```python
from build123d import *

# Parameters (mm, degrees)
SKETCH011_W     = 19.6
SKETCH011_H     = 4.05
PAD007_DEPTH    = 1.7
SKETCH005_R     = 3.1
PAD004_DEPTH    = 4.3
SKETCH004_R     = 3.1
PAD003_DEPTH    = 4.3
PAD_DEPTH       = 5.5
SKETCH001_W     = 89.8
SKETCH001_H     = 9.3
POCKET_DEPTH    = 3.75
SKETCH006_R     = 3.1
PAD005_DEPTH    = 4.2
SKETCH010_R     = 1.6
POCKET002_DEPTH = 3.2
SKETCH008_R     = 3.1
PAD006_DEPTH    = 4.2
SKETCH009_R     = 1.6
POCKET001_DEPTH = 3.2


with BuildPart() as body006:
    # Sketch011 → Pad007 (new body)
    with BuildSketch(Plane.YZ.offset(97.7)):
        with Locations((9.8, 3.725)):
            Rectangle(SKETCH011_W, SKETCH011_H)
    extrude(amount=-PAD007_DEPTH)


with BuildPart() as body002:
    # Sketch005 → Pad004 (new body)
    with BuildSketch(Plane.YZ.offset(93.4)):
        with Locations((20.07, 3.1)):
            Circle(SKETCH005_R)
    extrude(amount=PAD004_DEPTH)


with BuildPart() as fusion:
    # Sketch004 → Pad003 (new body)
    with BuildSketch(Plane.YZ):
        with Locations((20.07, 3.1)):
            Circle(SKETCH004_R)
    extrude(amount=PAD003_DEPTH)

    # Fusion: union Body002
    add(body002.part)


with BuildPart() as cut:
    # Sketch → Pad (new body)
    with BuildSketch(Plane.XY):
        Polygon((0, 0), (97.7, 0), (97.7, 20.1), (93.4, 20.1), (93.4, 15), (4.3, 15), (4.3, 20.1), (0, 20.1), align=None)
    extrude(amount=PAD_DEPTH)

    # Sketch001 (on Face10 of Pad) → Pocket (cut)
    with BuildSketch(Plane.XY.offset(5.5)):
        with Locations((48.9, 8.15)):
            Rectangle(SKETCH001_W, SKETCH001_H)
    extrude(amount=-POCKET_DEPTH, mode=Mode.SUBTRACT)

    # Cut: cut Fusion
    add(fusion.part, mode=Mode.SUBTRACT)


with BuildPart() as fusion001:
    # Sketch006 → Pad005 (new body)
    with BuildSketch(Plane.YZ):
        with Locations((20.07, 3.1)):
            Circle(SKETCH006_R)
    extrude(amount=PAD005_DEPTH)

    # Sketch010 (on Face2 of Pad005) → Pocket002 (cut)
    with BuildSketch(Plane(origin=(0, 0, 0), x_dir=(0, 1, 0), z_dir=(-1, 0, 0))):
        with Locations((20.07, -3.1)):
            Circle(SKETCH010_R)
    extrude(amount=-POCKET002_DEPTH, mode=Mode.SUBTRACT)

    # Fusion001: union Cut
    add(cut.part)


with BuildPart() as cut001:
    # Sketch008 → Pad006 (new body)
    with BuildSketch(Plane.YZ.offset(97.7)):
        with Locations((20.07, 3.1)):
            Circle(SKETCH008_R)
    extrude(amount=-PAD006_DEPTH)

    # Sketch009 (on Face2 of Pad006) → Pocket001 (cut)
    with BuildSketch(Plane.YZ.offset(97.7)):
        with Locations((20.07, 3.1)):
            Circle(SKETCH009_R)
    extrude(amount=-POCKET001_DEPTH, mode=Mode.SUBTRACT)

    # Fusion002: union Fusion001
    add(fusion001.part)

    # Cut001: cut Body006
    add(body006.part, mode=Mode.SUBTRACT)


solid = cut001.part
```
Read the model definition and answer for the solid it produces. Units are mm, in the model's axes. A direction names the side the tool comes from. Give positions to 0.01 mm unless a question says otherwise; leave off trailing zeros. Order: outer loops, then holes, each group sorted by start corner. A loop starts at its lowest first (then second) coordinate and runs counter-clockwise, first axis right, second up. Notation, with made-up numbers: (3.25, 52) -> (43.25, 52) arc R25 cw to (43.25, 68) -> close; hole circle Ø3 at (51, -32.5). An arc over 180 degrees is marked (long way). One line per item, written item: value. Start each with the question number.
(1) Straight lines are drawn through the part: L1, parallel to X at y = 19, z = 4.75; L2, parallel to X at y = 20.75, z = 5.25; L3, parallel to Z at x = 95.35, y = 20.07. For each, find the intervals that lie inside material, in ascending order.
(2) A tool of negligible diameter and unlimited length cuts with its end or side. For faces 1 (the flat face through (3.2, 20, 3)), 2 (the flat face through (49, 15, 3)), 3 (the flat face through (48, 3.5, 4)), from which of +Z, -Z, +X, -X, +Y, -Y can it reach the whole face along a straight path? Write none if from no direction.
(3) The part is cut by section C-C (y = 8.75). Determine the outline of the cut face in (x, z), and give its area (3 significant figures).
(4) The part is cut by section B-B (z = 3.1). Determine the outline of the cut face in (x, y).
(5) The part is cut by section A-A (y = 16). Determine the outline of the cut face in (x, z), and give its area (3 significant figures).
(6) The part is cut by section D-D (x = 78.5). Determine the outline of the cut face in (y, z), and give its area (3 significant figures).
(7) For a pull along Y with two mould halves and no side action, classify faces 4 (the cylindrical face through (2.07, 23.01, 4.08)), 5 (the flat face through (48, 3, 5.5)), 6 (the cylindrical face through (1.58, 18.47, 3.03)), 7 (the flat face through (4, 8, 4)) as released by +Y, released by -Y, zero draft, split by the parting line, or undercut.
(8) Flat-ended cylindrical pins translate along their axes: P1, Ø3, axis at y = 18.5, z = 2.5, coming from the +X side; P2, Ø1, axis at x = 14, z = 2, coming from the +Y side; P3, Ø1, axis at y = 19.5, z = 3.5, coming from the -X side; P4, Ø2, axis at x = 25, y = 11.5, coming from the +Z side. Find the tip coordinate at first contact, or state that the pin passes through.
Taken from the geometry:
1. L1: 0 to 4.2, 93.5 to 96
1. L2: 0 to 4.2, 93.5 to 97.7
1. L3: 0 to 1.5, 4.7 to 6.2
2. face 1: -X
2. face 2: +Z, -Z, +Y
2. face 3: +Z
3. outline: (0, 0) -> (97.7, 0) -> (97.7, 1.7) -> (96, 1.7) -> (96, 5.5) -> (93.8, 5.5) -> (93.8, 1.75) -> (4, 1.75) -> (4, 5.5) -> (0, 5.5) -> close
3. area: 194 mm^2
4. outline: (0, 0) -> (96, 0) -> (96, 18.47) -> (94.5, 18.47) -> (94.5, 21.67) -> (97.7, 21.67) -> (97.7, 23.17) -> (93.5, 23.17) -> (93.5, 16.97) -> (93.4, 16.97) -> (93.4, 15) -> (4.3, 15) -> (4.3, 16.97) -> (4.2, 16.97) -> (4.2, 23.17) -> (0, 23.17) -> (0, 21.67) -> (3.2, 21.67) -> (3.2, 18.47) -> (0, 18.47) -> close; hole (4, 3.5) -> (93.8, 3.5) -> (93.8, 12.8) -> (4, 12.8) -> close
5. outline: (0, 0) -> (4.3, 0) -> (4.3, 5.5) -> (0, 5.5) -> close; (93.4, 0) -> (97.7, 0) -> (97.7, 1.7) -> (96, 1.7) -> (96, 5.5) -> (93.4, 5.5) -> close
5. area: 40.8 mm^2
6. outline: (0, 0) -> (15, 0) -> (15, 5.5) -> (12.8, 5.5) -> (12.8, 1.75) -> (3.5, 1.75) -> (3.5, 5.5) -> (0, 5.5) -> close
6. area: 47.6 mm^2
7. face 4: split by the parting line
7. face 5: zero draft
7. face 6: undercut
7. face 7: undercut
8. P1: x = 97.7
8. P2: y = 15
8. P3: x = 3.2
8. P4: z = 1.75
